```python
from build123d import *

# Parameters (mm, degrees)
BOSS_EXTRUDE1_DEPTH      = 10
BOSS_EXTRUDE1_DEPTH_BACK = 10
SKETCH1_R                = 42.5
CUT_EXTRUDE6_REACH       = 194.75
CUT_EXTRUDE6_END_RADIUS  = 42.5
SKETCH3_R                = 3.5


with BuildPart() as part:
    # Sketch1 → Boss-Extrude1 (new, two sides: drawn at the far end of the back side and taken through both)
    with BuildSketch(Plane(origin=(0, 0, 0), x_dir=(1, 0, 0), z_dir=(0, 1, 0)).offset(-BOSS_EXTRUDE1_DEPTH_BACK)):
        with BuildLine():
            ThreePointArc((40, 30), (-50, 0), (40, -30))
            Line((40, -30), (238.383087675, -30))
            Line((238.383087675, -30), (238.383087675, 30))
            Line((238.383087675, 30), (40, 30))
        make_face()
        with Locations(Location((0, 0, 0), (0, 0, 270))):
            Circle(SKETCH1_R, mode=Mode.SUBTRACT)
    extrude(amount=BOSS_EXTRUDE1_DEPTH + BOSS_EXTRUDE1_DEPTH_BACK)

    # Cut-Extrude6: up to this cylinder (the profile starts outside it)
    cut_extrude6_end = Plane(origin=(0, 0, 0), z_dir=(0, 1, 0)) * Cylinder(CUT_EXTRUDE6_END_RADIUS, 475.5, mode=Mode.PRIVATE)
    # Sketch3 → Cut-Extrude6 (cut, up to the surface)
    with BuildSketch(Plane.ZY.offset(-52.5), mode=Mode.PRIVATE) as cut_extrude6_sk1:
        with Locations(Location((0, 0, 0), (0, 0, 180))):
            Circle(SKETCH3_R)
    cut_extrude6_tool1 = extrude(cut_extrude6_sk1.sketch, amount=CUT_EXTRUDE6_REACH, mode=Mode.PRIVATE) - cut_extrude6_end
    cut_extrude6 = cut_extrude6_tool1.solids().sort_by_distance((52.5, 0, 0))[0]
    add(cut_extrude6, mode=Mode.SUBTRACT)

    # Mirror1: Cut-Extrude6 across plane
    add(cut_extrude6.mirror(Plane(origin=(0, 0, 0), x_dir=(0, 0, 1), z_dir=(1, 0, 0))), mode=Mode.SUBTRACT)


solid = part.part
```
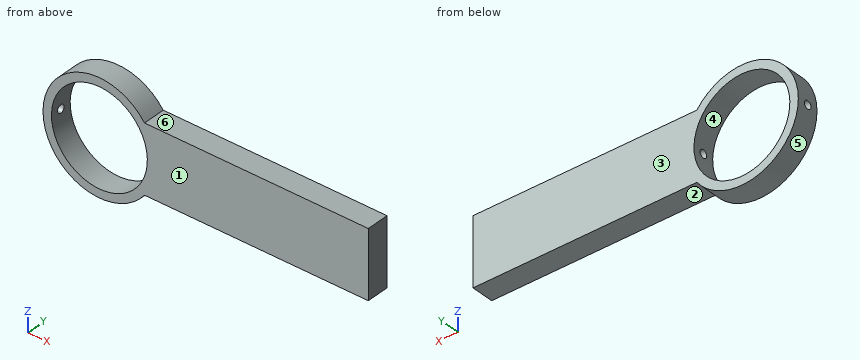
Geometry check sheet. Reference: the model listing, model coordinates, mm. Face numbers are marked on the shaded views. A direction names the side the tool comes from. Coordinates: 2 decimals unless noted, no trailing zeros. Order: outer loops, then holes, each group sorted by start corner. A loop starts at its lowest first (then second) coordinate and runs counter-clockwise, first axis right, second up. Notation, with made-up numbers: (-2.5, 28.5) - (43.5, 28.5) arc R34 ccw to (43.5, 61.5) - close; hole circle Ø10 at (-35, 18.25). An arc over 180 degrees is marked (long way). Use one line per item in the form item = value.
1. Section check B-B (x = 0). Record the boundary of the cut face in (y, z).
Here are the results:
outline = (-10, -50) - (10, -50) - (10, -42.5) - (-10, -42.5) - close; (-10, 42.5) - (10, 42.5) - (10, 50) - (-10, 50) - close
2. Section check D-D (y = 0). Record the boundary of the cut face in (x, z), then the cut area to 3 significant figures.
Here are the results:
outline = (-49.88, -3.5) arc R50 ccw to (40, -30) - (238.38, -30) - (238.38, 30) - (40, 30) arc R50 ccw to (-49.88, 3.5) - (-42.36, 3.5) arc R42.5 cw to (42.36, 3.5) - (52.5, 3.5) - (52.5, -3.5) - (42.36, -3.5) arc R42.5 cw to (-42.36, -3.5) - close
area = 13,600 mm²
3. Section check C-C (z = 35.5). Record the boundary of the cut face in (x, y).
Here are the results:
outline = (-35.21, -10) - (-23.37, -10) - (-23.37, 10) - (-35.21, 10) - close; (23.37, -10) - (35.21, -10) - (35.21, 10) - (23.37, 10) - close
4. Gauge pin test, flat ends, axial feed: pin 1 (1.5 mm diameter, centred on y = 2.5, z = -9.5, fed in from -X); pin 2 (4 mm diameter, centred on y = 0, z = 0, fed in from -X); pin 3 (6 mm diameter, centred on x = 125.5, y = 3, fed in from -Z). Record the tip position at first contact, or that the pin passes through.
Here are the results:
pin_1 = -49.23
pin_2 = 52.5
pin_3 = -30
5. Scan lines: line 1 (Y direction, x = 50, z = 0); line 2 (Z direction, x = 114.5, y = -8.5); line 3 (X direction, y = -7.5, z = 26.5). Record each from-to range of solid material in increasing order.
Here are the results:
line_1 = -10 to -3.5, 3.5 to 10
line_2 = -30 to 30
line_3 = -42.4 to -33.23, 33.23 to 238.38
6. Draft check along Z on the marked faces 3, 4, 5 and 6. Enter one of: pulls with the +Z half, pulls with the -Z half, needs draft (parallel to the pull), parting line crosses it, or undercut.
Here are the results:
face_3 = needs draft
face_4 = undercut
face_5 = parting line crosses it
face_6 = pulls with the +Z half
7. Access from +Z, -Z, +X, -X, +Y, -Y to the whole of each face (thin tool, end or side, straight path). Record for the marked faces 1 and 2.
Here are the results:
face_1 = +Z, -Z, +X, -X, -Y
face_2 = -Z, +X, +Y, -Y
8. Section check A-A (z = 0). Record the boundary of the cut face in (x, y).
Here are the results:
outline = (-50, -10) - (-42.5, -10) - (-42.5, -3.5) - (-50, -3.5) - close; (-50, 3.5) - (-42.5, 3.5) - (-42.5, 10) - (-50, 10) - close; (42.5, -10) - (238.38, -10) - (238.38, 10) - (42.5, 10) - (42.5, 3.5) - (52.5, 3.5) - (52.5, -3.5) - (42.5, -3.5) - close
